For this review, take the finished solid that the model builds, in its own axes (mm). Face numbers are marked on the shaded views. A direction names the side the tool comes from. Coordinates: 2 decimals unless noted, no trailing zeros. Order: outer loops, then holes, each group sorted by start corner. A loop starts at its lowest first (then second) coordinate and runs counter-clockwise, first axis right, second up. Notation, with made-up numbers: (-37, 59) -> (-14, 59) arc R22 cw to (-14, 79) -> close; hole circle Ø6 at (22.25, -19.75). An arc over 180 degrees is marked (long way). Write item = value, one per line. Start each with the question number.
1) Draft analysis for pull direction X (two halves, no side actions). For the marked faces 1, 2 and 3, state which applies: +X half, -X half, draft (parallel to the pull), parting line (faces both ways), or undercut.
2) Consider section A-A on y = 22.86. Give the boundary of the cut face in (x, z) (3 decimals).
3) Insertion check: pin 1 Ø3 at (x, y) = (2, 47.5) entering from -Z; pin 2 Ø5 at (y, z) = (49, 6.5) entering from +X. Each pin has a flat end and moves straight along its axis. Give the tip position at first contact, or say it passes through.
4) Wall thickness on probe 1 along Y at (x, z) = (18.5, 12); probe 2 along Y at (x, z) = (38.1, 4) (3 decimals): over which ranges is each line inside the solid? List them lowest first. Write a range as [from, to].
5) Consider section C-C on z = 3.5. Give the boundary of the cut face in (x, y) (3 decimals), and give its area (3 significant figures).
6) Consider section D-D on x = 48.5. Give the boundary of the cut face in (y, z), and give its area (3 significant figures).
7) Machinability: for the marked faces 4, 5, 6 and 7, which of the approach directions +Z, -Z, +X, -X, +Y, -Y give a long, thin tool a straight path to every point of the face, cutting with its end or side? Answer none if there is none.
8) Consider section B-B on x = 38.1. Give the boundary of the cut face in (y, z) (3 decimals).
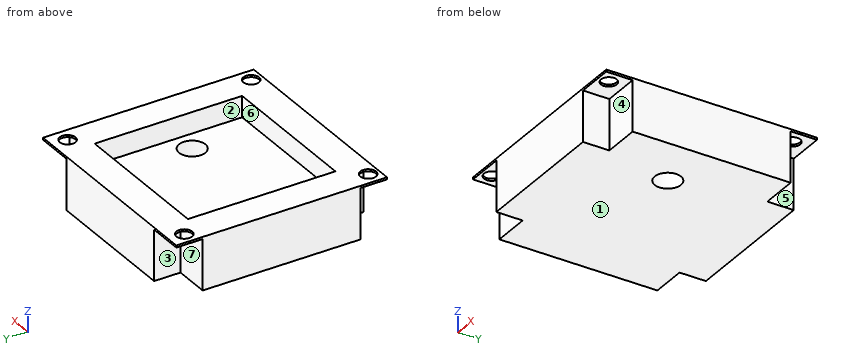
from build123d import *

# Parameters (mm, degrees)
SKETCH1_W           = 50.8
SKETCH1_H           = 50.8
BOSS_EXTRUDE1_DEPTH = 12.7
SHELL1_T            = -7.62
SKETCH3_W           = 8.89
SKETCH3_H           = 6.35
SKETCH3_W_2         = 8.455127559
CUT_EXTRUDE2_DEPTH  = 12.192
SKETCH4_R           = 1.905
CUT_EXTRUDE3_DEPTH  = 20.574
SKETCH6_R           = 3.175
CUT_EXTRUDE5_DEPTH  = 8.89


with BuildPart() as part:
    # Sketch1 → Boss-Extrude1 (new body)
    with BuildSketch(Plane.XY):
        with Locations((25.4, 25.4)):
            Rectangle(SKETCH1_W, SKETCH1_H)
    extrude(amount=BOSS_EXTRUDE1_DEPTH)

    # Shell1
    shell1_openings = [part.faces().sort_by_distance(p)[0] for p in [
        (25.4, 25.4, 12.7),
    ]]
    offset(amount=SHELL1_T, openings=shell1_openings, kind=Kind.INTERSECTION)

    # Sketch3 → Cut-Extrude2 (cut)
    with BuildSketch(Plane(origin=(0, 0, 0), x_dir=(-1, 0, 0), z_dir=(0, 0, -1))):
        with Locations((-46.355, 47.625)):
            Rectangle(SKETCH3_W, SKETCH3_H)
        with Locations((-46.355, 3.175)):
            Rectangle(SKETCH3_W, SKETCH3_H)
        with Locations((-4.445, 3.175)):
            Rectangle(SKETCH3_W, SKETCH3_H)
        with Locations((-4.22756378, 47.625)):
            Rectangle(SKETCH3_W_2, SKETCH3_H)
    extrude(amount=-CUT_EXTRUDE2_DEPTH, mode=Mode.SUBTRACT)

    # Sketch4 → Cut-Extrude3 (cut)
    with BuildSketch(Plane.XY.offset(12.7)):
        with Locations((2.97778213, 46.99)):
            Circle(SKETCH4_R)
        with Locations((47.42778213, 47.001802338)):
            Circle(SKETCH4_R)
        with Locations((3.166736342, 2.54)):
            Circle(SKETCH4_R)
        with Locations((47.616736342, 2.617819139)):
            Circle(SKETCH4_R)
    extrude(amount=-CUT_EXTRUDE3_DEPTH, mode=Mode.SUBTRACT)

    # Sketch6 → Cut-Extrude5 (cut)
    with BuildSketch(Plane(origin=(0, 0, 0), x_dir=(-1, 0, 0), z_dir=(0, 0, -1))):
        with Locations((-38.1, 22.86)):
            Circle(SKETCH6_R)
    extrude(amount=-CUT_EXTRUDE5_DEPTH, mode=Mode.SUBTRACT)


solid = part.part
Answer sheet:
q1.face_1 = draft
q1.face_2 = undercut
q1.face_3 = -X half
q2.outline = (0, 0) -> (34.925, 0) -> (34.925, 7.62) -> (7.62, 7.62) -> (7.62, 12.7) -> (0, 12.7) -> close; (41.275, 0) -> (50.8, 0) -> (50.8, 12.7) -> (43.18, 12.7) -> (43.18, 7.62) -> (41.275, 7.62) -> close
q3.pin_1 = 12.19
q3.pin_2 = 41.91
q4.probe_1 = [0, 7.62], [43.18, 50.8]
q4.probe_2 = [0, 19.685], [26.035, 50.8]
q5.outline = (0, 6.35) -> (8.89, 6.35) -> (8.89, 0) -> (41.91, 0) -> (41.91, 6.35) -> (50.8, 6.35) -> (50.8, 44.45) -> (41.91, 44.45) -> (41.91, 50.8) -> (8.455, 50.8) -> (8.455, 44.45) -> (0, 44.45) -> close; hole circle Ø6.35 at (38.1, 22.86)
q5.area = 2,330 mm2
q6.outline = (0, 12.19) -> (0.93, 12.19) -> (0.93, 12.7) -> (0, 12.7) -> close; (4.31, 12.19) -> (6.35, 12.19) -> (6.35, 0) -> (44.45, 0) -> (44.45, 12.19) -> (45.43, 12.19) -> (45.43, 12.7) -> (4.31, 12.7) -> close; (48.58, 12.19) -> (50.8, 12.19) -> (50.8, 12.7) -> (48.58, 12.7) -> close
q6.area = 487 mm2
q7.face_4 = -Z, +X, -Y
q7.face_5 = -Z, +X, +Y
q7.face_6 = +Z
q7.face_7 = -Z, -X, +Y
q8.outline = (0, 0) -> (19.685, 0) -> (19.685, 7.62) -> (7.62, 7.62) -> (7.62, 12.7) -> (0, 12.7) -> close; (26.035, 0) -> (50.8, 0) -> (50.8, 12.7) -> (43.18, 12.7) -> (43.18, 7.62) -> (26.035, 7.62) -> close
